from build123d import *

# Parameters (mm, degrees)
SKETCH_1_R          = 14.149308539
SKETCH_1_R_2        = 2.058081242
EXTRUDE_1_DEPTH     = 8
SKETCH_2_R          = 2.1
CUT_EXTRUDE_1_DEPTH = 37.249137921
SKETCH_3_R          = 11
CUT_EXTRUDE_2_DEPTH = 4


with BuildPart() as part:
    # 草图1 → 凸台-拉伸1 (new body)
    # profile 1 of 2: a face of its own
    with BuildSketch(Plane.XY):
        with BuildLine():
            ThreePointArc((20, 25), (23.535533906, 23.535533906), (25, 20))
            Line((25, 20), (25, -20))
            ThreePointArc((25, -20), (23.535533906, -23.535533906), (20, -25))
            Line((20, -25), (-20, -25))
            ThreePointArc((-20, -25), (-23.535533906, -23.535533906), (-25, -20))
            Line((-25, -20), (-25, 20))
            ThreePointArc((-25, 20), (-23.535533906, 23.535533906), (-20, 25))
            Line((-20, 25), (20, 25))
        make_face()
        Circle(SKETCH_1_R, mode=Mode.SUBTRACT)
    # profile 2 of 2: a face of its own
    with BuildSketch(Plane.XY):
        Circle(SKETCH_1_R)
        with Locations((-8, 0)):
            Circle(SKETCH_1_R_2, mode=Mode.SUBTRACT)
        with Locations((0, -8)):
            Circle(SKETCH_1_R_2, mode=Mode.SUBTRACT)
        with Locations((8, 0)):
            Circle(SKETCH_1_R_2, mode=Mode.SUBTRACT)
        with Locations((0, 8)):
            Circle(SKETCH_1_R_2, mode=Mode.SUBTRACT)
    extrude(amount=EXTRUDE_1_DEPTH)

    # 草图2 → 切除-拉伸1 (cut, through all)
    with BuildSketch(Plane.XY.offset(8)):
        with Locations((-15, 15)):
            Circle(SKETCH_2_R)
        with Locations(Location((-15, -15, 0), (0, 0, 180))):
            Circle(SKETCH_2_R)
        with Locations((15, -15)):
            Circle(SKETCH_2_R)
        with Locations(Location((15, 15, 0), (0, 0, 180))):
            Circle(SKETCH_2_R)
        with Locations(Location((21.213203436, 0, 0), (0, 0, 180))):
            Circle(SKETCH_2_R)
        with Locations((0, 21.213203436)):
            Circle(SKETCH_2_R)
        with Locations(Location((-21.213203436, 0, 0), (0, 0, 180))):
            Circle(SKETCH_2_R)
        with Locations((0, -21.213203436)):
            Circle(SKETCH_2_R)
    extrude(amount=-CUT_EXTRUDE_1_DEPTH, mode=Mode.SUBTRACT)

    # 草图3 → 切除-拉伸2 (cut)
    with BuildSketch(Plane.XY.offset(8)):
        Circle(SKETCH_3_R)
    extrude(amount=-CUT_EXTRUDE_2_DEPTH, mode=Mode.SUBTRACT)


solid = part.part
Work out the finished part from the listing and answer in its coordinate system (mm). A direction names the side the tool comes from. Round coordinates to 2 decimals unless told otherwise and drop trailing zeros. Write each loop counter-clockwise with the first axis right and the second up, starting at its lowest first coordinate (ties: lowest second). Pieces come first, ordered by that corner, then holes. Notation, with made-up numbers: (-15.75, -10) -> (23.25, -10) arc R20 ccw to (23.25, 21) -> close; hole circle Ø11 at (71, -30.5). An arc over 180 degrees is marked (long way). Answer as CSV lines item,"result". Start each with the question number.
(1) The part is cut by section D-D, the plane x = 8. Give the vertices of the cut face in (y, z), then the cut area to 3 significant figures.
(2) The part is cut by section A-A, the plane x = 15. Give the vertices of the cut face in (y, z), then the cut area to 3 significant figures.
(3) Find the intervals of material crossed by probe 1 along Y at (x, z) = (0, 4.25); probe 2 along X at (y, z) = (8, 1.8); probe 3 along X at (y, z) = (1, 5.75), in increasing order.
(4) A tool of negligible diameter and unlimited length cuts with its end or side. For faces 1 (the cylindrical face through (-19.115, -0.092, 4.056)), 2 (the flat face through (0, 0, 4)), from which of +Z, -Z, +X, -X, +Y, -Y can it reach the whole face along a straight path? Write none if from no direction.
(5) The mould has two halves that part along X. Classify faces 3 (the cylindrical face through (-1.52, -6.61, 1.97)), 4 (the cylindrical face through (14.727, -12.918, 4.056)), 5 (the flat face through (0, 25, 4)), 6 (the flat face through (25, 0, 4)): +X half, -X half, draft (parallel to the pull), parting line (faces both ways), or undercut.
(6) Each of these flat-tipped pins is pushed along its axis until it touches: pin 1 (6 mm diameter, centred on x = 0, y = 15.5, fed in from -Z); pin 2 (5.5 mm diameter, centred on x = -8, y = 0, fed in from +Z). Where does it stop, or does it pass through?
(7) The part is cut by section B-B, the plane y = 0. Give the vertices of the cut face in (x, z).
Output values:
1,outline,"(-25, 0) -> (-2.06, 0) -> (-2.06, 4) -> (-7.55, 4) -> (-7.55, 8) -> (-25, 8) -> close; (2.06, 0) -> (25, 0) -> (25, 8) -> (7.55, 8) -> (7.55, 4) -> (2.06, 4) -> close"
1,area,"323 mm²"
2,outline,"(-25, 0) -> (-17.1, 0) -> (-17.1, 8) -> (-25, 8) -> close; (-12.9, 0) -> (12.9, 0) -> (12.9, 8) -> (-12.9, 8) -> close; (17.1, 0) -> (25, 0) -> (25, 8) -> (17.1, 8) -> close"
2,area,"333 mm²"
3,probe 1,"y = -25 to -23.31, -19.11 to -11, 11 to 19.11, 23.31 to 25"
3,probe 2,"x = -25 to -2.06, 2.06 to 25"
3,probe 3,"x = -25 to -23.06, -19.37 to -10.95, 10.95 to 19.37, 23.06 to 25"
4,face 1,"+Z, -Z"
4,face 2,"+Z"
5,face 3,"undercut"
5,face 4,"undercut"
5,face 5,"draft"
5,face 6,"+X half"
6,pin 1,"stops at z = 0"
6,pin 2,"stops at z = 4"
7,outline,"(-25, 0) -> (-23.31, 0) -> (-23.31, 8) -> (-25, 8) -> close; (-19.11, 0) -> (-10.06, 0) -> (-10.06, 4) -> (-11, 4) -> (-11, 8) -> (-19.11, 8) -> close; (-5.94, 0) -> (5.94, 0) -> (5.94, 4) -> (-5.94, 4) -> close; (10.06, 0) -> (19.11, 0) -> (19.11, 8) -> (11, 8) -> (11, 4) -> (10.06, 4) -> close; (23.31, 0) -> (25, 0) -> (25, 8) -> (23.31, 8) -> close"
